Design review of the part built by this model. Coordinates are the model's own, in mm. Face numbers are marked on the shaded views. A direction names the side the tool comes from. Coordinates: 2 decimals unless noted, no trailing zeros. Loops run counter-clockwise (first coordinate to the right, second up) from the corner with the lowest first, then second, coordinate; pieces in that order, holes last. Notation, with made-up numbers: M 88.25,-20 L 144.25,-20 A21 cw 144.25,-2 Z; hole C 76,58.5 d8. An arc over 180 degrees is marked long. Write item = value, one per line. Start each with the question number.
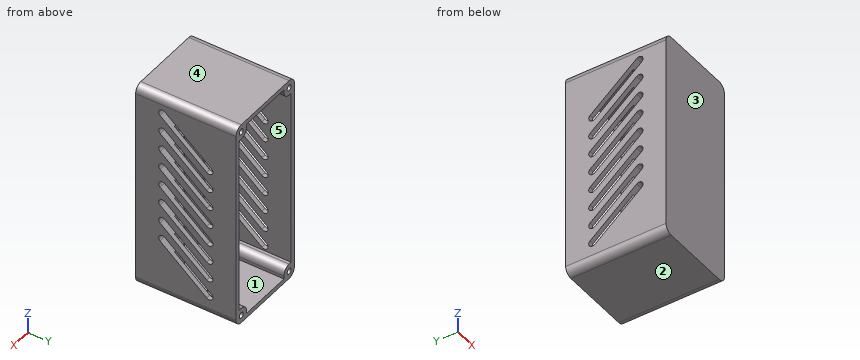
from build123d import *
from OCP.BRepFilletAPI import BRepFilletAPI_MakeFillet

# Parameters (mm, degrees)
SKETCH1_W               = 56
SKETCH1_H               = 138
BOSS_EXTRUDE1_DEPTH     = 65.95
SKETCH2_W               = 50
SKETCH2_H               = 132
CUT_EXTRUDE1_DEPTH      = 62.95
FILLET1_R1              = 2
FILLET1_R2              = 5
SKETCH3_R               = 1.9
BOSS_EXTRUDE2_DEPTH     = 62.95
MIRROR5_COPY_1_SKETCH_R = 1.9
MIRROR5_COPY_1_DEPTH    = 62.95
BOSS_EXTRUDE3_DEPTH     = 130
CUT_EXTRUDE2_DEPTH      = 74


with BuildPart() as part:
    # Sketch1 → Boss-Extrude1 (new body)
    with BuildSketch(Plane(origin=(0, 0, 0), x_dir=(1, 0, 0), z_dir=(0, 1, 0))):
        Rectangle(SKETCH1_W, SKETCH1_H)
    extrude(amount=BOSS_EXTRUDE1_DEPTH)

    # Sketch2 → Cut-Extrude1 (cut)
    with BuildSketch(Plane(origin=(0, 65.95, 0), x_dir=(1, 0, 0), z_dir=(0, 1, 0))):
        Rectangle(SKETCH2_W, SKETCH2_H)
    extrude(amount=-CUT_EXTRUDE1_DEPTH, mode=Mode.SUBTRACT)

    # Fillet1: one fillet with a radius per group of edges: ONE call of the kernel's fillet builder (fillet() takes one radius for all edges)
    fillet1_edges_1 = [part.edges().sort_by_distance(p)[0] for p in [
        (-25, 34.475, -66),
        (25, 34.475, -66),
        (-25, 34.475, 66),
        (25, 34.475, 66),
    ]]
    fillet1_edges_2 = [part.edges().sort_by_distance(p)[0] for p in [
        (-28, 32.975, -69),
        (28, 32.975, 69),
        (-28, 32.975, 69),
        (28, 32.975, -69),
    ]]
    fillet1 = BRepFilletAPI_MakeFillet(part.part.solid().wrapped)
    for e in fillet1_edges_1:
        fillet1.Add(FILLET1_R1, e.wrapped)
    for e in fillet1_edges_2:
        fillet1.Add(FILLET1_R2, e.wrapped)
    add(Compound.cast(fillet1.Shape()), mode=Mode.REPLACE)

    # Sketch3 → Boss-Extrude2 (add)
    with BuildSketch(Plane(origin=(0, 3, 0), x_dir=(1, 0, 0), z_dir=(0, 1, 0))):
        with BuildLine():
            Line((-23, 59), (-25, 59))
            Line((-25, 59), (-25, 64))
            ThreePointArc((-25, 64), (-24.414213562, 65.414213562), (-23, 66))
            Line((-23, 66), (-18, 66))
            Line((-18, 66), (-18, 64))
            ThreePointArc((-18, 64), (-19.464466094, 60.464466094), (-23, 59))
        make_face()
        with Locations(Location((-23, 64, 0), (0, 0, 90))):
            Circle(SKETCH3_R, mode=Mode.SUBTRACT)
    boss_extrude2 = extrude(amount=BOSS_EXTRUDE2_DEPTH)

    # Mirror4: Boss-Extrude2 across plane
    add(boss_extrude2.mirror(Plane.ZY))

    # Mirror5: Boss-Extrude2 across plane
    add(boss_extrude2.mirror(Plane.XY))

    # Mirror5 copy 1 sketch → Mirror5 copy 1 (add)
    with BuildSketch(Plane(origin=(0, 3, 0), x_dir=(-1, 0, 0), z_dir=(0, 1, 0))):
        with BuildLine():
            Line((-23, 59), (-25, 59))
            Line((-25, 59), (-25, 64))
            ThreePointArc((-25, 64), (-24.414213562, 65.414213562), (-23, 66))
            Line((-23, 66), (-18, 66))
            Line((-18, 66), (-18, 64))
            ThreePointArc((-18, 64), (-19.464466094, 60.464466094), (-23, 59))
        make_face()
        with Locations(Location((-23, 64, 0), (0, 0, 90))):
            Circle(MIRROR5_COPY_1_SKETCH_R, mode=Mode.SUBTRACT)
    extrude(amount=MIRROR5_COPY_1_DEPTH)

    # Sketch5 → Boss-Extrude3 (add)
    with BuildSketch(Plane(origin=(0, 0, 66), x_dir=(-1, 0, 0), z_dir=(0, 0, -1))):
        with BuildLine():
            ThreePointArc((0, 2.89979319), (-0.559053777, 2.942812119), (-1.116836261, 3))
            Line((-1.116836261, 3), (-18, 3))
            Line((-18, 3), (-18, 23.457091763))
            Line((-18, 23.457091763), (-26.3, 23.457091763))
            Line((-26.3, 23.457091763), (-26.3, 2.516966341))
            Line((-26.3, 2.516966341), (26.3, 2.516966341))
            Line((26.3, 2.516966341), (26.3, 23.457091763))
            Line((26.3, 23.457091763), (18, 23.457091763))
            Line((18, 23.457091763), (18, 3))
            Line((18, 3), (1.116836261, 3))
            ThreePointArc((1.116836261, 3), (0.559053777, 2.942812119), (0, 2.89979319))
        make_face()
        with BuildLine():
            Line((-18, 3), (-1.116836261, 3))
            ThreePointArc((-1.116836261, 3), (-6.149765384, 4.18974194), (-10.768389976, 6.516578486))
            ThreePointArc((-10.768389976, 6.516578486), (-14.0952442, 10.159119925), (-15.3, 14.942908237))
            Line((-15.3, 14.942908237), (-15.3, 23.457091763))
            Line((-15.3, 23.457091763), (-18, 23.457091763))
            Line((-18, 23.457091763), (-18, 3))
        make_face()
        with BuildLine():
            ThreePointArc((10.768389976, 6.516578486), (6.149765384, 4.18974194), (1.116836261, 3))
            Line((1.116836261, 3), (18, 3))
            Line((18, 3), (18, 23.457091763))
            Line((18, 23.457091763), (15.3, 23.457091763))
            Line((15.3, 23.457091763), (15.3, 14.942908237))
            ThreePointArc((15.3, 14.942908237), (14.0952442, 10.159119925), (10.768389976, 6.516578486))
        make_face()
    extrude(amount=BOSS_EXTRUDE3_DEPTH)

    # Sketch4 → Cut-Extrude2 (cut)
    with BuildSketch(Plane(origin=(28, 0, 0), x_dir=(0, 0, -1), z_dir=(1, 0, 0))):
        with BuildLine():
            Line((-59.770863302, 19.261080162), (-34.059358914, 49.902857887))
            ThreePointArc((-34.059358914, 49.902857887), (-30.537278782, 50.21099997), (-30.229136698, 46.688919838))
            Line((-30.229136698, 46.688919838), (-55.940641086, 16.047142113))
            ThreePointArc((-55.940641086, 16.047142113), (-59.462721218, 15.73900003), (-59.770863302, 19.261080162))
        make_face()
        with BuildLine():
            Line((-47.270863302, 19.261080162), (-21.559358914, 49.902857887))
            ThreePointArc((-21.559358914, 49.902857887), (-18.037278782, 50.21099997), (-17.729136698, 46.688919838))
            Line((-17.729136698, 46.688919838), (-43.440641086, 16.047142113))
            ThreePointArc((-43.440641086, 16.047142113), (-46.962721218, 15.73900003), (-47.270863302, 19.261080162))
        make_face()
        with BuildLine():
            Line((-34.770863302, 19.261080162), (-9.059358914, 49.902857887))
            ThreePointArc((-9.059358914, 49.902857887), (-5.537278782, 50.21099997), (-5.229136698, 46.688919838))
            Line((-5.229136698, 46.688919838), (-30.940641086, 16.047142113))
            ThreePointArc((-30.940641086, 16.047142113), (-34.462721218, 15.73900003), (-34.770863302, 19.261080162))
        make_face()
        with BuildLine():
            Line((-22.270863302, 19.261080162), (3.440641086, 49.902857887))
            ThreePointArc((3.440641086, 49.902857887), (6.962721218, 50.21099997), (7.270863302, 46.688919838))
            Line((7.270863302, 46.688919838), (-18.440641086, 16.047142113))
            ThreePointArc((-18.440641086, 16.047142113), (-21.962721218, 15.73900003), (-22.270863302, 19.261080162))
        make_face()
        with BuildLine():
            Line((-9.770863302, 19.261080162), (15.940641086, 49.902857887))
            ThreePointArc((15.940641086, 49.902857887), (19.462721218, 50.21099997), (19.770863302, 46.688919838))
            Line((19.770863302, 46.688919838), (-5.940641086, 16.047142113))
            ThreePointArc((-5.940641086, 16.047142113), (-9.462721218, 15.73900003), (-9.770863302, 19.261080162))
        make_face()
        with BuildLine():
            Line((2.729136698, 19.261080162), (28.440641086, 49.902857887))
            ThreePointArc((28.440641086, 49.902857887), (31.962721218, 50.21099997), (32.270863302, 46.688919838))
            Line((32.270863302, 46.688919838), (6.559358914, 16.047142113))
            ThreePointArc((6.559358914, 16.047142113), (3.037278782, 15.73900003), (2.729136698, 19.261080162))
        make_face()
        with BuildLine():
            Line((15.229136698, 19.261080162), (40.940641086, 49.902857887))
            ThreePointArc((40.940641086, 49.902857887), (44.462721218, 50.21099997), (44.770863302, 46.688919838))
            Line((44.770863302, 46.688919838), (19.059358914, 16.047142113))
            ThreePointArc((19.059358914, 16.047142113), (15.537278782, 15.73900003), (15.229136698, 19.261080162))
        make_face()
        with BuildLine():
            Line((27.729136698, 19.261080162), (53.440641086, 49.902857887))
            ThreePointArc((53.440641086, 49.902857887), (56.962721218, 50.21099997), (57.270863302, 46.688919838))
            Line((57.270863302, 46.688919838), (31.559358914, 16.047142113))
            ThreePointArc((31.559358914, 16.047142113), (28.037278782, 15.73900003), (27.729136698, 19.261080162))
        make_face()
    extrude(amount=-CUT_EXTRUDE2_DEPTH, mode=Mode.SUBTRACT)


solid = part.part
Q1. Mouldability with a two-part tool opening along Z and no side actions: class the marked faces 1, 2 and 3 as released by +Z, released by -Z, zero draft, split by the parting line, or undercut.
Q2. To check wall thickness, follow line 1 (Z direction, x = 23, y = 46); line 2 (X direction, y = 51, z = 64); line 3 (Z direction, x = 6, y = 28). State the ranges of each line that lie inside material, in increasing order. Write a range as from..to.
Q3. Add section C-C on x = 2.5. State the section outline as (y, z) points.
Q4. Add section D-D on x = -6. State the section outline as (y, z) points, plus the area to 3 significant figures.
Q5. Add section B-B on z = -42.5. Give the number of separate pieces and of enclosed holes in the cut face, plus the area to 3 significant figures.
Q6. For the marked faces 4 and 5, list the 3-axis set-ups (+Z, -Z, +X, -X, +Y, -Y) from which the entire face can be reached by the end or side of a thin tool; tool diameter is ignored.
Q7. Clearance check with flat-ended pins moving along their axes: P1, Ø1.8, axis at x = 20.5, z = -2.5, coming from the +Y side; P2, Ø12, axis at x = 11.5, z = 49.5, coming from the -Y side; P3, Ø1.6, axis at x = -24, y = 52, coming from the +Z side; P4, Ø4, axis at x = -9.5, z = 15.5, coming from the +Y side. State where each tip first meets the part, or that it passes through.
Q8. Add section A-A on y = 54. State the section outline as (x, z) points.
Values follow:
q1.face_1 = undercut
q1.face_2 = released by -Z
q1.face_3 = zero draft
q2.line_1 = -69..-65.9, -62.1..-59, 59..62.1, 65.9..69
q2.line_2 = -28..-24.9, -21.1..-18, 18..21.1, 24.9..28
q2.line_3 = -69..-66, 66..69
q3.outline = M 0,-69 L 65.95,-69 L 65.95,-66 L 3,-66 L 3,-64 L 3.2,-64 L 3.2,66 L 65.95,66 L 65.95,69 L 0,69 Z
q4.outline = M 0,-69 L 65.95,-69 L 65.95,-66 L 3,-66 L 3,-64 L 4.14,-64 L 4.14,66 L 65.95,66 L 65.95,69 L 0,69 Z
q4.area = 939 mm2
q5.separate_pieces = 5
q5.enclosed_holes = 0
q5.area = 935 mm2
q6.face_4 = +Z, +X, -X, +Y, -Y
q6.face_5 = +Y
q7.P1 = 23.46
q7.P2 = 0
q7.P3 = 69
q7.P4 = 7.05
q8.outline = M -28,-64 A5 ccw -23,-69 L 23,-69 A5 ccw 28,-64 L 28,64 A5 ccw 23,69 L -23,69 A5 ccw -28,64 Z; hole M -25,-59 L -23,-59 A5 cw -18,-64 L -18,-66 L 18,-66 L 18,-64 A5 cw 23,-59 L 25,-59 L 25,59 L 23,59 A5 cw 18,64 L 18,66 L -18,66 L -18,64 A5 cw -23,59 L -25,59 Z; hole C -23,-64 d3.8; hole C -23,64 d3.8; hole C 23,-64 d3.8; hole C 23,64 d3.8
